Geometry: final body of the model. Coordinates: model frame, mm. Face numbers are marked on the shaded views. Coordinates: 2 decimals unless noted, no trailing zeros. Order: outer loops, then holes, each group sorted by start corner. A loop starts at its lowest first (then second) coordinate and runs counter-clockwise, first axis right, second up. Notation, with made-up numbers: (10, -5) - (34, -5) arc R21 cw to (34, 28) - close; hole circle Ø7 at (-27, 68.5). An arc over 180 degrees is marked (long way). Use a Markdown table: item, result. Add a question column.
Autodesk Inventor part; units mm, degrees
ref_plane "YZ Plane" through (0, 0, 0) normal (1, 0, 0) x (0, 1, 0)
ref_plane "XZ Plane" through (0, 0, 0) normal (0, 1, 0) x (-1, 0, 0)
ref_plane "XY Plane" through (0, 0, 0) normal (0, 0, 1) x (1, 0, 0)
sketch "Sketch1" plane through (0, 0, 0) normal (0, 0, 1) x (1, 0, 0)
  line L0 (13.4938, 0) -> (6.7469, -11.6859)
  line L1 (6.7469, -11.6859) -> (-6.7469, -11.6859)
  line L2 (-6.7469, -11.6859) -> (-13.4938, 0)
  line L3 (-13.4938, 0) -> (-6.7469, 11.6859)
  line L4 (-6.7469, 11.6859) -> (6.7469, 11.6859)
  line L5 (6.7469, 11.6859) -> (13.4938, 0)
  circle A0 centre (0, 0) radius 7.1755
  point P0 (0, 0)
  point P1 (0, 0)
  dimension "d0" = 26.9875
  dimension "d1" = 14.351
extrude "Extrusion1" add sketch "Sketch1" along normal blind 7.62
fillet "Fillet1" radius 0.3175 18 edges at (0, 11.6859, 7.62) (6.7469, 11.6859, 3.81) (-6.7469, 11.6859, 3.81) (0, 11.6859, 0) (10.1203, 5.843, 7.62) (10.1203, 5.843, 0) (13.4938, 0, 3.81) (10.1203, -5.843, 0) (10.1203, -5.843, 7.62) (6.7469, -11.6859, 3.81) (0, -11.6859, 7.62) (0, -11.6859, 0) (-6.7469, -11.6859, 3.81) (-10.1203, -5.843, 0) (-10.1203, -5.843, 7.62) (-13.4938, 0, 3.81) (-10.1203, 5.843, 7.62) (-10.1203, 5.843, 0)
thread "Thread1"
properties part number "Large Nut" material "Stainless Steel"
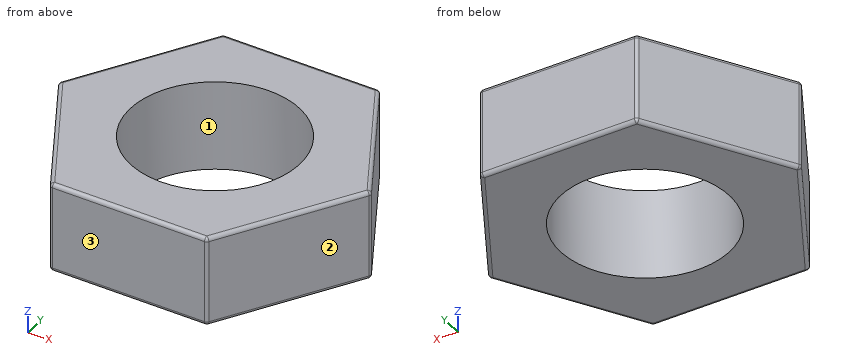
1) Draft query along X for the marked faces 1, 2 and 3. Return one class per face: pulls with the +X half, pulls with the -X half, needs draft (parallel to the pull), parting line crosses it, or undercut.
2) Pin query (flat end, axial travel): pin 1 (4 mm diameter, centred on y = -7.5, z = 6, fed in from +X); pin 2 (1.5 mm diameter, centred on y = 1, z = 3.5, fed in from -X); pin 3 (3 mm diameter, centred on y = 7.5, z = 4, fed in from +X). Return the tip coordinate at first contact, or that it passes through.
3) Section B-B (x = 0). Return loops of the section in (y, z) (1 decimal), then the cut area to 3 significant figures.
4) Ray query, line 1 along Y through (x, z) = (0, 5); line 2 along X through (y, z) = (5, 2); line 3 along Y through (x, z) = (5.25, 3.75). Return the intervals inside material, ascending.
Values follow:
| question | item | result |
|---|---|---|
| 1 | face 1 | undercut |
| 1 | face 2 | pulls with the +X half |
| 1 | face 3 | needs draft |
| 2 | pin 1 | stops at x = 10.32 |
| 2 | pin 2 | stops at x = -13.35 |
| 2 | pin 3 | stops at x = 10.03 |
| 3 | outline | (-11.7, 0.3) arc R0.3 ccw to (-11.4, 0) - (-7.2, 0) - (-7.2, 7.6) - (-11.4, 7.6) arc R0.3 ccw to (-11.7, 7.3) - close; (7.2, 0) - (11.4, 0) arc R0.3 ccw to (11.7, 0.3) - (11.7, 7.3) arc R0.3 ccw to (11.4, 7.6) - (7.2, 7.6) - close |
| 3 | area | 68.7 mm² |
| 4 | line 1 | y = -11.69 to -7.18, 7.18 to 11.69 |
| 4 | line 2 | x = -10.61 to -5.15, 5.15 to 10.61 |
| 4 | line 3 | y = -11.69 to -4.89, 4.89 to 11.69 |
